Can you work these out from the drawing? Everything is in mm from the part's minimum corner. A direction names the side the tool comes from. Round coordinates to 2 decimals unless told otherwise and drop trailing zeros. Order: outer loops, then holes, each group sorted by start corner. A loop starts at its lowest first (then second) coordinate and runs counter-clockwise, first axis right, second up. Notation, with made-up numbers: M 10.25,49.5 L 23.25,49.5 A16 cw 23.25,55.5 Z; hole C -38,-5.75 d5. An arc over 180 degrees is marked long. Answer as CSV lines item,"result". Start each with the question number.
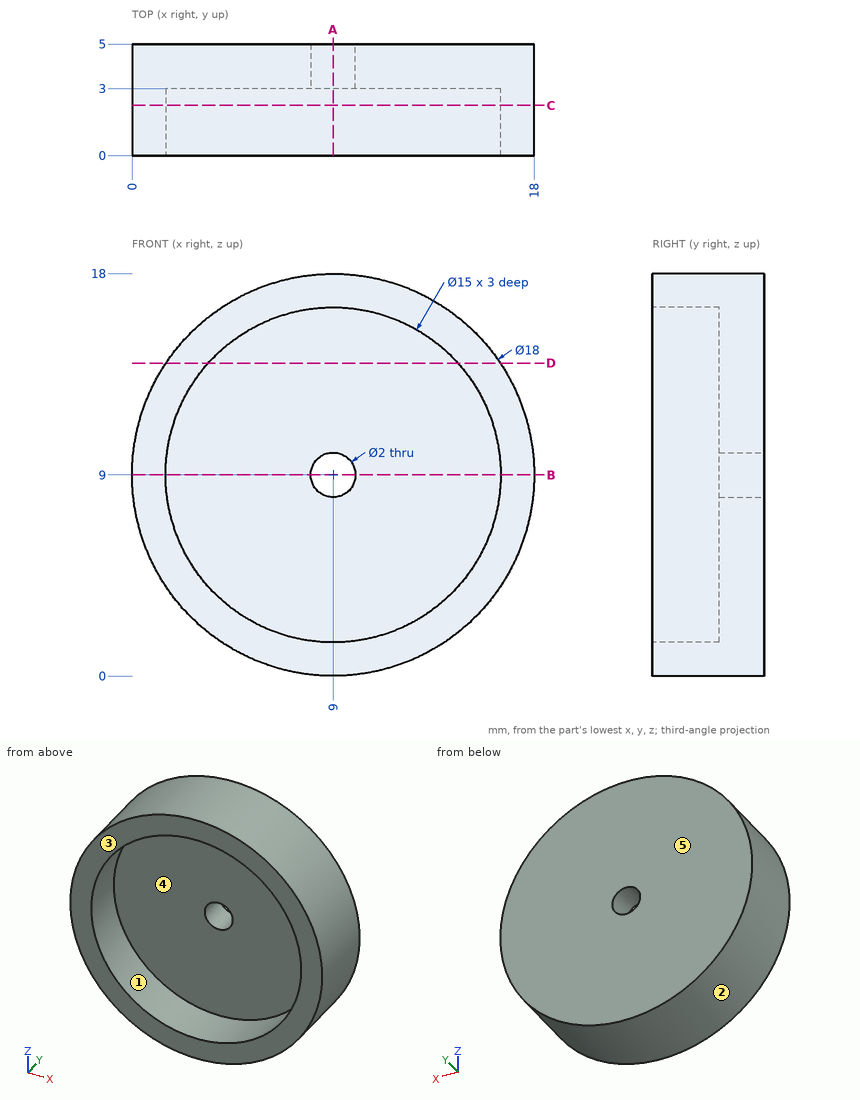
(1) I want a section at B-B on z = 9. Write out the boundary of the cut face in (x, y).
(2) I'm going to push flat-ended pins straight in: P1, Ø2, axis at x = 4.5, y = 1, coming from the +Z side; P2, Ø7.5, axis at x = 11.5, z = 8.5, coming from the -Y side; P3, Ø1, axis at y = 3.5, z = 6.5, coming from the -X side. Where does each tip first touch, or does it pass through?
(3) I want a section at C-C on y = 2.25. Write out the boundary of the cut face in (x, z).
(4) I want a section at A-A on x = 9. Write out the boundary of the cut face in (y, z), and give its area (3 significant figures).
(5) If we mould it in two halves opening along Z, with no side actions, what happens to the marked faces 1, 2 and 3? For each: +Z half, -Z half, draft (parallel to the pull), parting line (faces both ways), or undercut.
(6) I want a section at D-D on z = 14. Write out the boundary of the cut face in (x, y).
(7) For the marked faces 4 and 5, which set-ups out of +Z, -Z, +X, -X, +Y, -Y let a thin tool reach every point of the face, with its end or its side?
(8) If I drill on line 1 along X through (y, z) = (2.25, 9); line 2 along Z through (x, y) = (9, 4.4), over which ranges is the centre line in solid material (lowest first)?
From the geometry:
1,outline,"M 0,0 L 1.5,0 L 1.5,3 L 8,3 L 8,5 L 0,5 Z; M 10,3 L 16.5,3 L 16.5,0 L 18,0 L 18,5 L 10,5 Z"
2,P1,"z = 17.29"
2,P2,"y = 3"
2,P3,"x = 0.23"
3,outline,"C 9,9 d18; hole C 9,9 d15"
4,outline,"M 0,0 L 5,0 L 5,8 L 3,8 L 3,1.5 L 0,1.5 Z; M 0,16.5 L 3,16.5 L 3,10 L 5,10 L 5,18 L 0,18 Z"
4,area,"41.0 mm²"
5,face 1,"undercut"
5,face 2,"parting line"
5,face 3,"draft"
6,outline,"M 1.52,0 L 3.41,0 L 3.41,3 L 14.59,3 L 14.59,0 L 16.48,0 L 16.48,5 L 1.52,5 Z"
7,face 4,"-Y"
7,face 5,"+Z, -Z, +X, -X, +Y"
8,line 1,"0 to 1.5, 16.5 to 18"
8,line 2,"0 to 8, 10 to 18"
